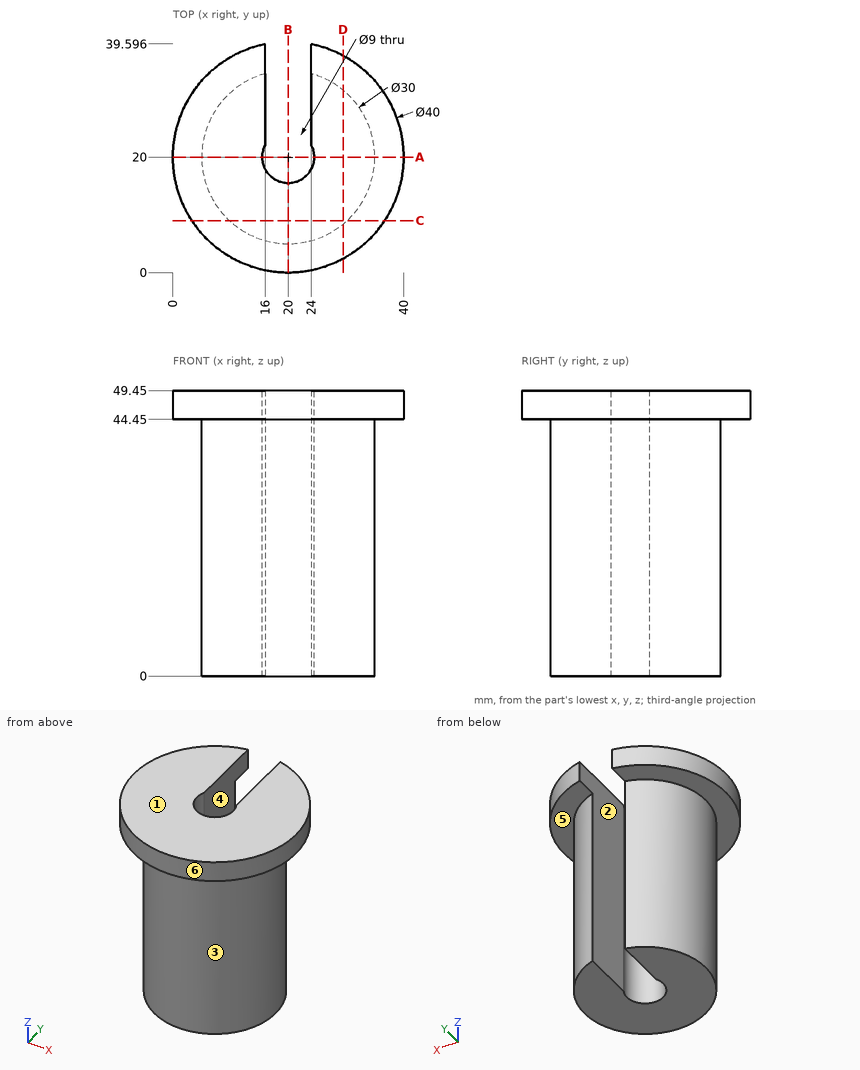
Answer from the drawing. Dimensions are ordinates in mm from the lowest x, y and z of the part. A direction names the side the tool comes from. Coordinates: 2 decimals unless noted, no trailing zeros. Order: outer loops, then holes, each group sorted by start corner. A loop starts at its lowest first (then second) coordinate and runs counter-clockwise, first axis right, second up. Notation, with made-up numbers: M -23.5,77 L 35.5,77 A25 cw 35.5,107 Z; hole C 38,84.5 d11. An arc over 180 degrees is marked long. Put each result on its own line as item: value. Start each with the question number.
Item 1: Section B-B, the plane x = 20 is taken. Determine the outline of the cut face in (y, z), plus the area to 3 significant figures.
Item 2: Consider probe 1 along X at (y, z) = (20, 30); probe 2 along Z at (x, y) = (8, 7.5); probe 3 along X at (y, z) = (25.5, 41.5) (1 decimal). Determine where each line is inside the solid, lowest interval first. Write a range as [from, to].
Item 3: For the marked faces 4, 5 and 6, determine the directions among +Z, -Z, +X, -X, +Y, -Y from which every point of the face is accessible in a straight line to the end or side of a thin tool.
Item 4: Section A-A, the plane y = 20 is taken. Determine the outline of the cut face in (x, z), plus the area to 3 significant figures.
Item 5: Section D-D, the plane x = 29.5 is taken. Determine the outline of the cut face in (y, z), plus the area to 3 significant figures.
Item 6: The mould has two halves that part along X. Classify the marked faces 1, 2 and 3: +X half, -X half, draft (parallel to the pull), parting line (faces both ways), or undercut.
Item 7: Section C-C, the plane y = 9 is taken. Determine the outline of the cut face in (x, z), plus the area to 3 significant figures.
Item 8: Given pin 1 Ø3 at (x, z) = (20, 11) entering from +Y; pin 2 Ø6 at (y, z) = (27.5, 10.5) entering from -X; pin 3 Ø5.5 at (y, z) = (33, 13) entering from +X; pin 4 Ø5.5 at (x, y) = (20, 20) entering from +Z (3 decimals), each flat-ended and moving along its own axis, determine where each tip first touches the part or whether it passes through.
Computed:
1. outline: M 0,44.45 L 5,44.45 L 5,0 L 15.5,0 L 15.5,49.45 L 0,49.45 Z
1. area: 544 mm2
2. probe 1: x = [5, 15.5], [24.5, 35]
2. probe 2: z = [44.45, 49.45]
2. probe 3: x = [6, 16], [24, 34]
3. face 4: +Z, -Z, +Y
3. face 5: -Z
3. face 6: +Z, -Z
4. outline: M 0,44.45 L 5,44.45 L 5,0 L 15.5,0 L 15.5,49.45 L 0,49.45 Z; M 24.5,0 L 35,0 L 35,44.45 L 40,44.45 L 40,49.45 L 24.5,49.45 Z
4. area: 1,090 mm2
5. outline: M 2.4,44.45 L 8.39,44.45 L 8.39,0 L 31.61,0 L 31.61,44.45 L 37.6,44.45 L 37.6,49.45 L 2.4,49.45 Z
5. area: 1,210 mm2
6. face 1: draft
6. face 2: undercut
6. face 3: parting line
7. outline: M 3.3,44.45 L 9.8,44.45 L 9.8,0 L 30.2,0 L 30.2,44.45 L 36.7,44.45 L 36.7,49.45 L 3.3,49.45 Z
7. area: 1,070 mm2
8. pin 1: stops at y = 15.76
8. pin 2: stops at x = 5.69
8. pin 3: stops at x = 30.95
8. pin 4: passes through
